from build123d import *

# Parameters (mm, degrees)
SKETCH1_R           = 35
SKETCH1_R_2         = 5
BOSS_EXTRUDE1_DEPTH = 10


with BuildPart() as part:
    # Sketch1 → Boss-Extrude1 (new body)
    with BuildSketch(Plane(origin=(0, 0, 0), x_dir=(1, 0, 0), z_dir=(0, 1, 0))):
        with BuildLine():
            ThreePointArc((-37.777777778, -13.146843962), (0, -40), (37.777777778, -13.146843962))
            ThreePointArc((37.777777778, -13.146843962), (39.954124614, -10.486884629), (43.333333333, -9.860132972))
            ThreePointArc((43.333333333, -9.860132972), (55, 0), (43.333333333, 9.860132972))
            ThreePointArc((43.333333333, 9.860132972), (39.954124614, 10.486884629), (37.777777778, 13.146843962))
            ThreePointArc((37.777777778, 13.146843962), (0, 40), (-37.777777778, 13.146843962))
            ThreePointArc((-37.777777778, 13.146843962), (-39.954124614, 10.486884629), (-43.333333333, 9.860132972))
            ThreePointArc((-43.333333333, 9.860132972), (-55, 0), (-43.333333333, -9.860132972))
            ThreePointArc((-43.333333333, -9.860132972), (-39.954124614, -10.486884629), (-37.777777778, -13.146843962))
        make_face()
        with Locations(Location((0, 0, 0), (0, 0, 270))):
            Circle(SKETCH1_R, mode=Mode.SUBTRACT)
        with Locations(Location((-45, 0, 0), (0, 0, 270))):
            Circle(SKETCH1_R_2, mode=Mode.SUBTRACT)
        with Locations(Location((45, 0, 0), (0, 0, 270))):
            Circle(SKETCH1_R_2, mode=Mode.SUBTRACT)
    extrude(amount=BOSS_EXTRUDE1_DEPTH)


solid = part.part
Could you check a few things on this model? Use its own coordinates, in mm. Give positions to 0.01 mm unless a question says otherwise; leave off trailing zeros. Write each loop counter-clockwise with the first axis right and the second up, starting at its lowest first coordinate (ties: lowest second). Pieces come first, ordered by that corner, then holes. Notation, with made-up numbers: (48.5, 89) -> (77.5, 89) arc R15 cw to (77.5, 106) -> close; hole circle Ø4 at (55, 64.5). An arc over 180 degrees is marked (long way). Answer as CSV lines item,"result". Start each with the question number.
(1) If we section it at D-D, the plane z = -23: Write out the boundary of the cut face in (x, y), and give its area (3 significant figures).
(2) If we section it at B-B, the plane z = 0: Write out the boundary of the cut face in (x, y).
(3) Please list where these lines run through material, in increasing order: line 1 (X direction, y = 2, z = -23.5); line 2 (Z direction, x = 9, y = 6.5); line 3 (X direction, y = 9.75, z = -32).
(4) If we mould it in two halves opening along X, with no side actions, what happens to faces 1 (the face through (-0.3, 0, 35.4)), 2 (the face through (39.912, 4.93, 10.512)), 3 (the face through (0.692, 4.93, -39.994))? For each: +X half, -X half, draft (parallel to the pull), parting line (faces both ways), or undercut.
(5) If we section it at A-A, the plane x = -45: Write out the boundary of the cut face in (y, z).
(6) I'm going to push flat-ended pins straight in: pin 1 Ø5 at (x, y) = (0.5, 7.5) entering from +Z; pin 2 Ø3 at (y, z) = (1.5, -22.5) entering from -X; pin 3 Ø13 at (x, z) = (-45, 0) entering from +Y; pin 4 Ø4 at (y, z) = (2, -24) entering from -X. Where does each tip first touch, or does it pass through?
(7) If we section it at C-C, the plane y = 5.5: Write out the boundary of the cut face in (x, z), and give its area (3 significant figures).
Answer list:
1,outline,"(-32.73, 0) -> (-26.38, 0) -> (-26.38, 10) -> (-32.73, 10) -> close; (26.38, 0) -> (32.73, 0) -> (32.73, 10) -> (26.38, 10) -> close"
1,area,"127 mm^2"
2,outline,"(-55, 0) -> (-50, 0) -> (-50, 10) -> (-55, 10) -> close; (-40, 0) -> (-35, 0) -> (-35, 10) -> (-40, 10) -> close; (35, 0) -> (40, 0) -> (40, 10) -> (35, 10) -> close; (50, 0) -> (55, 0) -> (55, 10) -> (50, 10) -> close"
3,line 1,"-32.37 to -25.94, 25.94 to 32.37"
3,line 2,"-38.97 to -33.82, 33.82 to 38.97"
3,line 3,"-24 to -14.18, 14.18 to 24"
4,face 1,"draft"
4,face 2,"undercut"
4,face 3,"parting line"
5,outline,"(0, -10) -> (10, -10) -> (10, -5) -> (0, -5) -> close; (0, 5) -> (10, 5) -> (10, 10) -> (0, 10) -> close"
6,pin 1,"z = 40"
6,pin 2,"x = -34.04"
6,pin 3,"y = 10"
6,pin 4,"x = -33.41"
7,outline,"(-43.33, -9.86) arc R5 cw to (-37.78, -13.15) arc R40 ccw to (37.78, -13.15) arc R5 cw to (43.33, -9.86) arc R10 ccw (long way) to (43.33, 9.86) arc R5 cw to (37.78, 13.15) arc R40 ccw to (-37.78, 13.15) arc R5 cw to (-43.33, 9.86) arc R10 ccw (long way) to start; hole circle Ø10 at (-45, 0); hole circle Ø70 at (0, 0); hole circle Ø10 at (45, 0)"
7,area,"1,560 mm^2"
